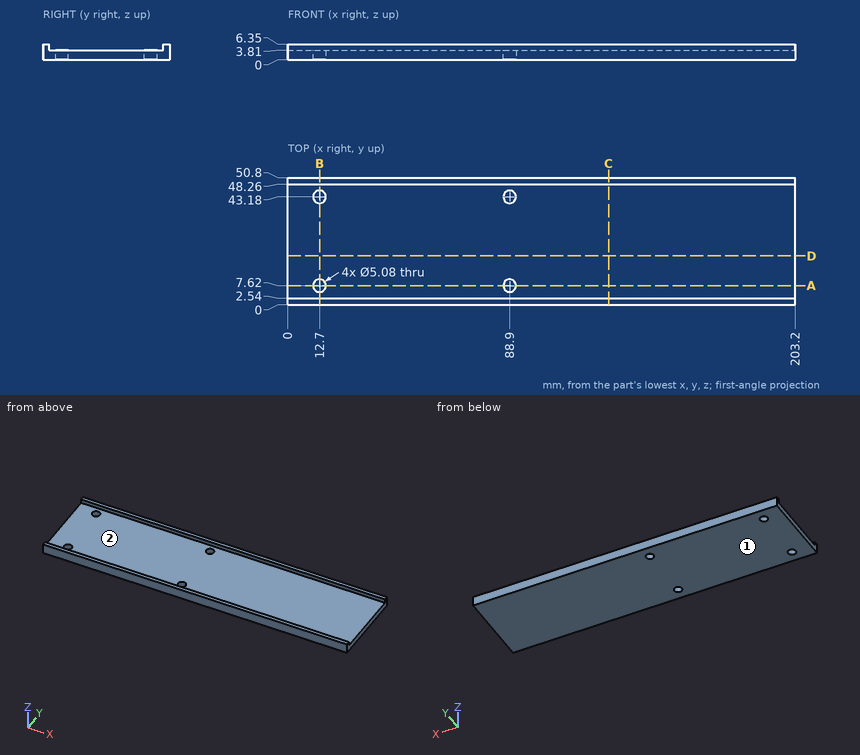
Could you check a few things on this drawing? It's one solid part, dimensions in mm from its lowest x, y, z. Give positions to 0.01 mm unless a question says otherwise; leave off trailing zeros. Order: outer loops, then holes, each group sorted by start corner. A loop starts at its lowest first (then second) coordinate and runs counter-clockwise, first axis right, second up. Notation, with made-up numbers: (-32.5, -18.5) - (-24.5, -18.5) arc R26 cw to (-24.5, 1.5) - close; hole circle Ø11 at (-31, 14). An arc over 180 degrees is marked (long way). Answer as a JSON object with one key per item and string values. Group by question number.
Item 1: If we section it at B-B on x = 12.7: Please give me the cut outline in (y, z).
Item 2: If we mould it in two halves opening along Y, with no side actions, what happens to the marked faces 1 and 2? For each: pulls with the +Y half, pulls with the -Y half, needs draft (parallel to the pull), parting line crosses it, or undercut.
Item 3: If we section it at C-C on x = 128.5: Please give me the cut outline in (y, z), and give its area (3 significant figures).
Item 4: For P1, Ø23, axis at x = 105, y = 15, coming from the +Z side; P2, Ø4.5, axis at x = 88.9, y = 7.62, coming from the -Z side, each with a flat end and sliding along its axis, tell me the tip position at first contact or that it passes through.
Item 5: If we section it at A-A on y = 7.62: Please give me the cut outline in (x, z).
Item 6: Please list where these lines run through material, in increasing order: probe 1 along Y at (x, z) = (88.9, 2.2); probe 2 along X at (y, z) = (43.5, 3.5); probe 3 along Y at (x, z) = (163.5, 5).
Item 7: If we section it at D-D on y = 19.5: Please give me the cut outline in (x, z).
Result set:
{
 "1": {"outline": "(0, 0) - (5.08, 0) - (5.08, 3.81) - (2.54, 3.81) - (2.54, 6.35) - (0, 6.35) - close; (10.16, 0) - (40.64, 0) - (40.64, 3.81) - (10.16, 3.81) - close; (45.72, 0) - (50.8, 0) - (50.8, 6.35) - (48.26, 6.35) - (48.26, 3.81) - (45.72, 3.81) - close"},
 "2": {"face 1": "needs draft", "face 2": "undercut"},
 "3": {"outline": "(0, 0) - (50.8, 0) - (50.8, 6.35) - (48.26, 6.35) - (48.26, 3.81) - (2.54, 3.81) - (2.54, 6.35) - (0, 6.35) - close", "area": "206 mm²"},
 "4": {"P1": "z = 3.81", "P2": "through"},
 "5": {"outline": "(0, 0) - (10.16, 0) - (10.16, 3.81) - (0, 3.81) - close; (15.24, 0) - (86.36, 0) - (86.36, 3.81) - (15.24, 3.81) - close; (91.44, 0) - (203.2, 0) - (203.2, 3.81) - (91.44, 3.81) - close"},
 "6": {"probe 1": "0 to 5.08, 10.16 to 40.64, 45.72 to 50.8", "probe 2": "0 to 10.18, 15.22 to 86.38, 91.42 to 203.2", "probe 3": "0 to 2.54, 48.26 to 50.8"},
 "7": {"outline": "(0, 0) - (203.2, 0) - (203.2, 3.81) - (0, 3.81) - close"}
}
